Build history of the part. All positions in model axes, mm. A direction names the side the tool comes from. Round coordinates to 2 decimals unless told otherwise and drop trailing zeros. Loops run counter-clockwise (first coordinate to the right, second up) from the corner with the lowest first, then second, coordinate; pieces in that order, holes last. Notation, with made-up numbers: M 25,68 L 83,68 A22 cw 83,106 Z; hole C 3,2.25 d10. An arc over 180 degrees is marked long. Use one line per item in the form item = value. Start each with the question number.
```python
from build123d import *

# Parameters (mm, degrees)
SKETCH1_R           = 2.525
BOSS_EXTRUDE1_DEPTH = 15.5
SKETCH2_R           = 4
BOSS_EXTRUDE2_DEPTH = 6
CUT_EXTRUDE1_START  = -5
CUT_EXTRUDE1_DEPTH  = 5
FILLET2_R           = 0.25
FILLET3_R           = 0.25
CUT_EXTRUDE2_DEPTH  = 11.5


with BuildPart() as part:
    # Sketch1 → Boss-Extrude1 (new body)
    with BuildSketch(Plane.XY):
        Circle(SKETCH1_R)
    extrude(amount=BOSS_EXTRUDE1_DEPTH)

    # Sketch2 → Boss-Extrude2 (add)
    with BuildSketch(Plane.XY.offset(15.5)):
        Circle(SKETCH2_R)
    extrude(amount=BOSS_EXTRUDE2_DEPTH)

    # Sketch3 → Cut-Extrude1 (cut)
    with BuildSketch(Plane.XY.offset(21.5).offset(CUT_EXTRUDE1_START)):
        with BuildLine():
            Line((-2.01246118, 1.525), (2.01246118, 1.525))
            ThreePointArc((2.01246118, 1.525), (2.525, 0), (2.01246118, -1.525))
            Line((2.01246118, -1.525), (-2.01246118, -1.525))
            ThreePointArc((-2.01246118, -1.525), (-2.525, 0), (-2.01246118, 1.525))
        make_face()
    extrude(amount=CUT_EXTRUDE1_DEPTH, mode=Mode.SUBTRACT)

    # Fillet2
    fillet2_edges = [part.edges().sort_by_distance(p)[0] for p in [
        (-4, 0, 21.5),
    ]]
    fillet(fillet2_edges, radius=FILLET2_R)

    # Fillet3
    fillet3_edges = [part.edges().sort_by_distance(p)[0] for p in [
        (-2.525, 0, 0),
    ]]
    fillet(fillet3_edges, radius=FILLET3_R)

    # Sketch4 → Cut-Extrude2 (cut)
    with BuildSketch(Plane(origin=(0, 0, 0), x_dir=(-1, 0, 0), z_dir=(0, 0, -1))):
        with BuildLine():
            Line((-2.25, 1.145916664), (2.25, 1.145916664))
            ThreePointArc((2.25, 1.145916664), (0, 2.525), (-2.25, 1.145916664))
        make_face()
    extrude(amount=-CUT_EXTRUDE2_DEPTH, mode=Mode.SUBTRACT)


solid = part.part
```
Q1. Saw through at B-B (x = 0). Give the cut face in (y, z) (3 decimals), and give its area (3 significant figures).
Q2. Saw through at D-D (z = 7.75). Give the cut face in (x, y) (3 decimals), and give its area (3 significant figures).
Q3. Pull direction X, two halves, no side cores. Call faces 5 (the face through (0, -1, 0)), 6 (the face through (0, 1.525, 19)), 7 (the face through (1.165, -2.24, 7.768)): pulls with the +X half, pulls with the -X half, needs draft (parallel to the pull), parting line crosses it, or undercut.
Q4. Saw through at C-C (z = 13.75). Give the cut face in (x, y) (3 decimals), and give its area (3 significant figures).
Q5. Tool access for faces 1 (the face through (0, 1.146, 6)), 2 (the face through (2.525, 0.023, 18.965)), 3 (the face through (3, 0, 15.5)), 4 (the face through (-0.867, -3.905, 18.335)): list every direction of +Z, -Z, +X, -X, +Y, -Y with a clear straight run to the whole face (end or side of a thin tool).
Q6. Wall check: probe 1 along Y at (x, z) = (0, 18.5) (3 decimals); probe 2 along Z at (x, y) = (0, 0.25); probe 3 along Y at (x, z) = (-1.5, 17) (3 decimals). Give the ranges that are in metal, low to high.
Q7. Drop flat-ended pins along their axis: P1, Ø1.5, axis at y = 0, z = 9, coming from the -X side (3 decimals); P2, Ø1.5, axis at x = -0.5, y = 2, coming from the -Z side; P3, Ø3, axis at y = 0.5, z = 12, coming from the +X side (3 decimals). Give the stop position or say it passes through.
Q8. Saw through at A-A (y = 0). Give the cut face in (x, z) (3 decimals), and give its area (3 significant figures).
Filled in:
q1.outline = M -4,15.5 L -2.525,15.5 L -2.525,0.25 A0.25 ccw -2.275,0 L 1.146,0 L 1.146,11.5 L 2.525,11.5 L 2.525,15.5 L 4,15.5 L 4,21.25 A0.25 ccw 3.75,21.5 L 1.525,21.5 L 1.525,16.5 L -1.525,16.5 L -1.525,21.5 L -3.75,21.5 A0.25 ccw -4,21.25 Z
q1.area = 95.1 mm²
q2.outline = M -2.25,1.146 A2.525 ccw long 2.25,1.146 Z
q2.area = 15.6 mm²
q3.face_5 = needs draft
q3.face_6 = undercut
q3.face_7 = parting line crosses it
q4.outline = C 0,0 d5.05
q4.area = 20.0 mm²
q5.face_1 = -Z, +X, -X, +Y
q5.face_2 = +Z
q5.face_3 = -Z
q5.face_4 = +Z, -Z
q6.probe_1 = -4 to -1.525, 1.525 to 4
q6.probe_2 = 0 to 16.5
q6.probe_3 = -3.708 to -1.525, 1.525 to 3.708
q7.P1 = -2.525
q7.P2 = 11.5
q7.P3 = 2.525
q8.outline = M -4,15.5 L -2.525,15.5 L -2.525,0.25 A0.25 ccw -2.275,0 L 2.275,0 A0.25 ccw 2.525,0.25 L 2.525,15.5 L 4,15.5 L 4,21.25 A0.25 ccw 3.75,21.5 L 2.525,21.5 L 2.525,16.5 L -2.525,16.5 L -2.525,21.5 L -3.75,21.5 A0.25 ccw -4,21.25 Z
q8.area = 101 mm²
